```python
from build123d import *

# Parameters (mm, degrees)
SKETCH1_W                  = 7.9375
SKETCH1_H                  = 12.7
BOSS_EXTRUDE1_DEPTH        = 3.175
SKETCH1_3_W                = 3.175
SKETCH1_3_H                = 12.7
BOSS_EXTRUDE2_DEPTH        = 12.7
CUT_EXTRUDE2_DEPTH         = 21.143116845
BOSS_EXTRUDE3_DEPTH        = 3.175
SKETCH4_W                  = 3.175
SKETCH4_H                  = 6.35
BOSS_EXTRUDE4_DEPTH        = 4.7625
SKETCH5_R                  = 0.1984375
CUT_EXTRUDE3_DEPTH         = 23.11131639
CHAMFER1_SIZE              = 0.4
CHAMFER2_SIZE              = 1
F_35_0_11_DIAMETER_HOLE1_D = 2.794
CHAMFER3_SIZE              = 0.2


with BuildPart() as part:
    # Sketch1 → Boss-Extrude1 (new body)
    with BuildSketch(Plane(origin=(0, 0, 0), x_dir=(1, 0, 0), z_dir=(0, 1, 0))):
        Rectangle(SKETCH1_W, SKETCH1_H)
    extrude(amount=BOSS_EXTRUDE1_DEPTH)

    # Sketch1<3> → Boss-Extrude2 (add)
    with BuildSketch(Plane(origin=(0, 0, 0), x_dir=(1, 0, 0), z_dir=(0, 1, 0))):
        with Locations((5.55625, 0)):
            Rectangle(SKETCH1_3_W, SKETCH1_3_H)
        with Locations((-5.55625, 0)):
            Rectangle(SKETCH1_3_W, SKETCH1_3_H)
    extrude(amount=BOSS_EXTRUDE2_DEPTH)

    # Sketch2 → Cut-Extrude2 (cut, through all)
    with BuildSketch(Plane(origin=(7.14375, 0, 0), x_dir=(0, 0, -1), z_dir=(1, 0, 0))):
        Polygon((-6.35, 3.175), (0, 12.7), (-6.35, 12.7), align=None)
    extrude(amount=-CUT_EXTRUDE2_DEPTH, mode=Mode.SUBTRACT)

    # Sketch3 → Boss-Extrude3 (add)
    with BuildSketch(Plane(origin=(0, 3.175, 0), x_dir=(1, 0, 0), z_dir=(0, 1, 0))):
        Polygon((-3.148, 3.148), (-3.148, 6.35), (-3.96875, 6.35), (-3.96875, -3.148), (-3.148, -3.148), align=None)
        Polygon((3.148, 3.148), (3.148, -3.148), (3.96875, -3.148), (3.96875, 6.35), (3.148, 6.35), align=None)
    extrude(amount=BOSS_EXTRUDE3_DEPTH)

    # Sketch4 → Boss-Extrude4 (add)
    with BuildSketch(Plane(origin=(0, 0, -6.35), x_dir=(-1, 0, 0), z_dir=(0, 0, -1))):
        with Locations((-5.55625, 6.35)):
            Rectangle(SKETCH4_W, SKETCH4_H)
        with Locations((5.55625, 6.35)):
            Rectangle(SKETCH4_W, SKETCH4_H)
    extrude(amount=BOSS_EXTRUDE4_DEPTH)

    # Sketch5 → Cut-Extrude3 (cut, through all)
    with BuildSketch(Plane(origin=(7.14375, 0, 0), x_dir=(0, 0, -1), z_dir=(1, 0, 0))):
        with Locations((6.35, 9.525)):
            Circle(SKETCH5_R)
        with Locations((6.35, 3.175)):
            Circle(SKETCH5_R)
    extrude(amount=-CUT_EXTRUDE3_DEPTH, mode=Mode.SUBTRACT)

    # Chamfer1
    chamfer1_edges = [part.edges().sort_by_distance(p)[0] for p in [
        (-5.55625, 9.525, -11.1125),
        (-5.55625, 3.175, -11.1125),
        (5.55625, 3.175, -11.1125),
        (5.55625, 9.525, -11.1125),
        (3.96875, 6.35, -1.601),
        (-3.96875, 6.35, -1.601),
    ]]
    chamfer(chamfer1_edges, length=CHAMFER1_SIZE)

    # Chamfer2
    chamfer2_edges = [part.edges().sort_by_distance(p)[0] for p in [
        (-7.14375, 12.7, -3.175),
        (7.14375, 12.7, -3.175),
        (7.14375, 7.9375, 3.175),
        (-7.14375, 7.9375, 3.175),
        (-7.14375, 1.5875, 6.35),
        (7.14375, 1.5875, 6.35),
        (0, 0, 6.35),
    ]]
    chamfer(chamfer2_edges, length=CHAMFER2_SIZE)

    # #35 (0.11) Diameter Hole1 (through all)
    with Locations(Plane(origin=(0, 3.175, 0), x_dir=(1, 0, 0), z_dir=(0, 1, 0))):
        with Locations((0, 0)):
            Hole(F_35_0_11_DIAMETER_HOLE1_D / 2)

    # Chamfer3
    chamfer3_edges = [part.edges().sort_by_distance(p)[0] for p in [
        (1.397, 3.175, 0),
        (1.397, 0, 0),
    ]]
    chamfer(chamfer3_edges, length=CHAMFER3_SIZE)


solid = part.part
```
Can you work these out from the model? Positions are in its coordinate system, mm. A direction names the side the tool comes from. Coordinates: 2 decimals unless noted, no trailing zeros. Loops run counter-clockwise (first coordinate to the right, second up) from the corner with the lowest first, then second, coordinate; pieces in that order, holes last. Notation, with made-up numbers: M 16,-13.75 L 52,-13.75 A9 cw 52,-0.75 Z; hole C 1.5,15 d11. An arc over 180 degrees is marked long. Put each result on its own line as item: value. Start each with the question number.
(1) Will these pins go through, and if not, where does the flat tip stop? pin 1 Ø3 at (x, z) = (-3.5, -8) entering from -Y (3 decimals); pin 2 Ø2 at (x, z) = (-2.5, 2.5) entering from -Y; pin 3 Ø1 at (x, z) = (-5, -8) entering from +Y (3 decimals); pin 4 Ø3 at (x, y) = (-4, 5) entering from +Z.
(2) Which directions (+Z, -Z, +X, -X, +Y, -Y) give clear straight access to the entire face, cutting with the end or side of a thin tool? Please do faces 1 (the face through (5, 12.7, -3)), 2 (the face through (-3.148, 5, -2)), 3 (the face through (0, 1, -6.35)), 4 (the face through (-6, 9.525, -9)).
(3) Imagine slicing it at A-A on z = -7. List the corners of the cut face in (x, y) for me (3 decimals).
(4) I need wall thicknesses on probe 1 along X at (y, z) = (3.5, -5); probe 2 along X at (y, z) = (5, -9.5); probe 3 along Y at (x, z) = (-3.75, -6.25). Which ranges of each line are inside material? Lowest first, please.
(5) Imagine slicing it at B-B on x = 0. List the corners of the cut face in (y, z) for me (3 decimals).
(6) Imagine slicing it at D-D on y = 11.25. List the corners of the cut face in (x, z) for me.
(7) We'd pull the mould along Z, two halves only. Please class faces 5 (the face through (0, 0, -2)), 6 (the face through (1.11, 1.57, 0.85)), 7 (the face through (-3.6, 5, -6.35)): +Z half, -Z half, draft (parallel to the pull), parting line (faces both ways), or undercut.
Worked answers:
1. pin 1: stops at y = 3.175
1. pin 2: stops at y = 0
1. pin 3: stops at y = 9.525
1. pin 4: stops at z = 6.13
2. face 1: +Z, -Z, +X, -X, +Y
2. face 2: +Z, -Z, +Y
2. face 3: -Z, +X, -X, -Y
2. face 4: -Z, +X, -X, +Y
3. outline: M -7.144,3.175 L -3.969,3.175 L -3.969,9.525 L -7.144,9.525 Z; M 3.969,3.175 L 7.144,3.175 L 7.144,9.525 L 3.969,9.525 Z
4. probe 1: x = -7.14 to -3.15, 3.15 to 7.14
4. probe 2: x = -7.14 to -3.97, 3.97 to 7.14
4. probe 3: y = 0 to 3, 3.35 to 6.53
5. outline: M 0,-6.35 L 2.977,-6.35 A0.198 cw 3.175,-6.152 L 3.175,-1.597 L 2.975,-1.397 L 0.2,-1.397 L 0,-1.597 Z; M 0,1.597 L 0.2,1.397 L 2.975,1.397 L 3.175,1.597 L 3.175,6.35 L 1,6.35 L 0,5.35 Z
6. outline: M -7.14,-6.35 L -3.97,-6.35 L -3.97,0.97 L -6.14,0.97 L -7.14,-0.24 Z; M 3.97,-6.35 L 7.14,-6.35 L 7.14,-0.24 L 6.14,0.97 L 3.97,0.97 Z
7. face 5: draft
7. face 6: undercut
7. face 7: -Z half
